Can you work these out from the drawing? Everything is in mm from the part's minimum corner. Round coordinates to 2 decimals unless told otherwise and drop trailing zeros. Write each loop counter-clockwise with the first axis right and the second up, starting at its lowest first coordinate (ties: lowest second). Pieces come first, ordered by that corner, then holes. Notation, with made-up numbers: M -1,-11.5 L 3,-11.5 A10 cw 3,-6.5 Z; hole C -18.75,57 d3. An arc over 180 degrees is marked long. Use one line per item in the form item = value. Start each with the question number.
Q1. I need wall thicknesses on line 1 along Y through (x, z) = (78.5, 0.4); line 2 along Y through (x, z) = (95, 1.9); line 3 along X through (y, z) = (59.5, 2.6). Which ranges of each line are inside material? Lowest first, please. Write a range as from..to.
Q2. I want a section at A-A on x = 20. List the corners of the cut face in (y, z) for me, and give its area (3 significant figures).
Q3. I want a section at D-D on z = 1.25. State how many separate pieces and enclosed holes the cut face has, and give its area (3 significant figures).
Q4. I want a section at C-C on x = 95. List the corners of the cut face in (y, z) for me, and give its area (4 significant figures).
Q5. I want a section at B-B on y = 41.25. List the corners of the cut face in (x, z) for me, and give its area (3 significant figures).
Q6. We'd pull the mould along Z, two halves only. Please class the marked faces 1 and 2: +Z half, -Z half, draft (parallel to the pull), parting line (faces both ways), or undercut.
Q7. I'm going to push a flat-ended pin straight in: pin 1 Ø3 at (x, y) = (95, 78.75) entering from -Z. Where does the tip first touch, or does it pass through?
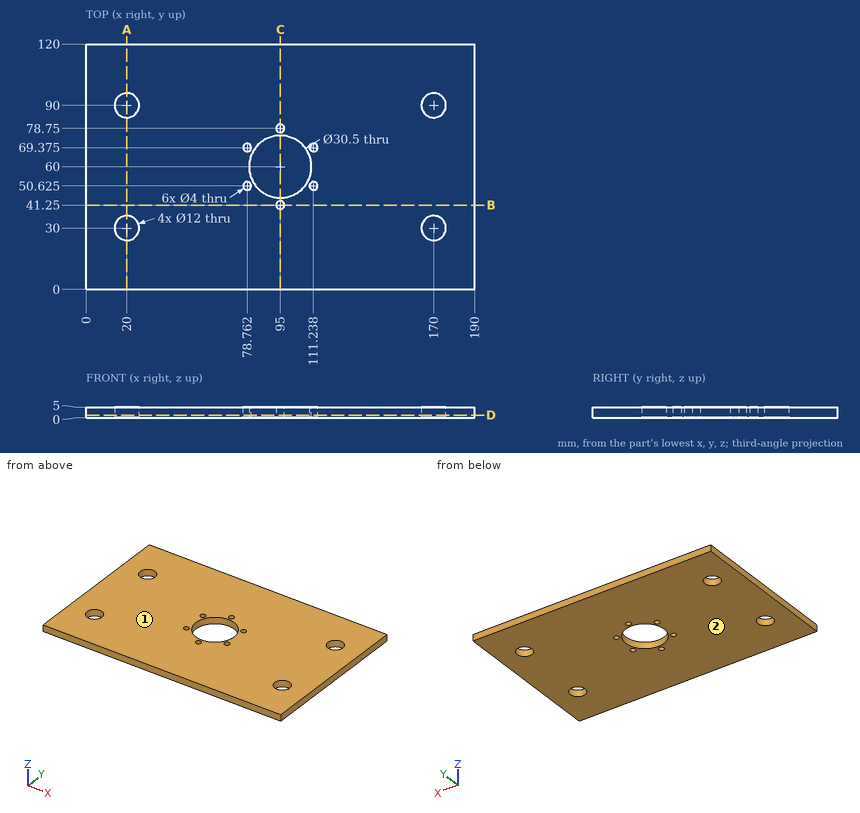
Reported:
q1.line_1 = 0..48.64, 52.61..67.39, 71.36..120
q1.line_2 = 0..39.25, 43.25..44.75, 75.25..76.75, 80.75..120
q1.line_3 = 0..79.76, 110.24..190
q2.outline = M 0,0 L 24,0 L 24,5 L 0,5 Z; M 36,0 L 84,0 L 84,5 L 36,5 Z; M 96,0 L 120,0 L 120,5 L 96,5 Z
q2.area = 480 mm^2
q3.separate_pieces = 1
q3.enclosed_holes = 11
q3.area = 21,500 mm^2
q4.outline = M 0,0 L 39.25,0 L 39.25,5 L 0,5 Z; M 43.25,0 L 44.75,0 L 44.75,5 L 43.25,5 Z; M 75.25,0 L 76.75,0 L 76.75,5 L 75.25,5 Z; M 80.75,0 L 120,0 L 120,5 L 80.75,5 Z
q4.area = 407.5 mm^2
q5.outline = M 0,0 L 93,0 L 93,5 L 0,5 Z; M 97,0 L 190,0 L 190,5 L 97,5 Z
q5.area = 930 mm^2
q6.face_1 = +Z half
q6.face_2 = -Z half
q7.pin_1 = through
